from build123d import *

# Parameters (mm, degrees)
BOSS_EXTRUDE1_DEPTH = 64
SKETCH2_R           = 2
CUT_EXTRUDE1_DEPTH  = 5.7
CUT_EXTRUDE2_START  = -5.7
SKETCH3_R           = 2
CUT_EXTRUDE2_DEPTH  = 5.7


with BuildPart() as part:
    # Sketch1 → Boss-Extrude1 (new body)
    with BuildSketch(Plane(origin=(0, 0, 0), x_dir=(1, 0, 0), z_dir=(0, 1, 0))):
        Polygon((-19.5, 39.5), (-19.5, -39.5), (12.5, -39.5), (12.5, -32.5), (-12.5, -32.5), (-12.5, 32.5), (12.5, 32.5), (12.5, 39.5), align=None)
    extrude(amount=BOSS_EXTRUDE1_DEPTH)

    # Sketch2 → Cut-Extrude1 (cut)
    with BuildSketch(Plane(origin=(0, 0, 0), x_dir=(1, 0, 0), z_dir=(0, 1, 0))):
        with Locations(Location((-16, 36, 0), (0, 0, 270))):
            Circle(SKETCH2_R)
        with Locations(Location((-16, -36, 0), (0, 0, 90))):
            Circle(SKETCH2_R)
        with Locations(Location((9, 36, 0), (0, 0, 270))):
            Circle(SKETCH2_R)
        with Locations(Location((9, -36, 0), (0, 0, 90))):
            Circle(SKETCH2_R)
    extrude(amount=CUT_EXTRUDE1_DEPTH, mode=Mode.SUBTRACT)

    # Sketch3 → Cut-Extrude2 (cut)
    with BuildSketch(Plane(origin=(0, 64, 0), x_dir=(1, 0, 0), z_dir=(0, 1, 0)).offset(CUT_EXTRUDE2_START)):
        with Locations(Location((-16, 0, 0), (0, 0, 270))):
            Circle(SKETCH3_R)
        with Locations(Location((9, -36, 0), (0, 0, 90))):
            Circle(SKETCH3_R)
        with Locations(Location((9, 36, 0), (0, 0, 270))):
            Circle(SKETCH3_R)
    extrude(amount=CUT_EXTRUDE2_DEPTH, mode=Mode.SUBTRACT)


solid = part.part
Read the model definition and answer for the solid it produces. Units are mm, in the model's axes. A direction names the side the tool comes from. Round coordinates to 2 decimals unless told otherwise and drop trailing zeros. Order: outer loops, then holes, each group sorted by start corner. A loop starts at its lowest first (then second) coordinate and runs counter-clockwise, first axis right, second up. Notation, with made-up numbers: (73.5, 19.25) - (85.5, 19.25) arc R28 ccw to (85.5, 56.25) - close; hole circle Ø8 at (20, 73). An arc over 180 degrees is marked (long way). Use one line per item in the form item = value. Start each with the question number.
(1) The part is cut by section C-C (z = -36). Give the vertices of the cut face in (x, y).
(2) Find the intervals of material crossed by line 1 along X through (y, z) = (3.5, 36); line 2 along Z through (x, y) = (8.5, 19.5); line 3 along X through (y, z) = (62.8, 0), in increasing order. Write a range as from..to.
(3) Flat-ended cylindrical pins translate along their axes: pin 1 Ø1.5 at (y, z) = (27, 31.5) entering from +X; pin 2 Ø2 at (x, z) = (9, -35.5) entering from +Y; pin 3 Ø3.5 at (x, z) = (9, -36) entering from -Y. Find the tip coordinate at first contact, or state that the pin passes through.
(4) The part is cut by section A-A (x = 9). Give the vertices of the cut face in (y, z), then the cut area to 3 significant figures.
(5) Determine the mould class of faces 5 (the face through (9, 58.3, -36)), 6 (the face through (-19.5, 32, -1)), 7 (the face through (-18, 64, -1)) for opening direction X: +X half, -X half, draft (parallel to the pull), parting line (faces both ways), or undercut.
(6) The part is cut by section B-B (y = 40.5). Give the vertices of the cut face in (x, z).
(7) The part is cut by section D-D (x = -4.5). Give the vertices of the cut face in (y, z).
(8) For faces 1 (the face through (9, 5.7, -36)), 2 (the face through (-12.5, 32, 0)), 3 (the face through (-4, 32, 39.5)), 4 (the face through (-14, 61, 0)), determine the directions among +Z, -Z, +X, -X, +Y, -Y from which every point of the face is accessible in a straight line to the end or side of a thin tool.
Checked values:
q1.outline = (-19.5, 0) - (-18, 0) - (-18, 5.7) - (-14, 5.7) - (-14, 0) - (7, 0) - (7, 5.7) - (11, 5.7) - (11, 0) - (12.5, 0) - (12.5, 64) - (11, 64) - (11, 58.3) - (7, 58.3) - (7, 64) - (-19.5, 64) - close
q2.line_1 = -19.5..-18, -14..7, 11..12.5
q2.line_2 = -39.5..-32.5, 32.5..39.5
q2.line_3 = -19.5..-18, -14..-12.5
q3.pin_1 = -12.5
q3.pin_2 = 58.3
q3.pin_3 = 5.7
q4.outline = (0, -39.5) - (64, -39.5) - (64, -38) - (58.3, -38) - (58.3, -34) - (64, -34) - (64, -32.5) - (0, -32.5) - (0, -34) - (5.7, -34) - (5.7, -38) - (0, -38) - close; (0, 32.5) - (64, 32.5) - (64, 34) - (58.3, 34) - (58.3, 38) - (64, 38) - (64, 39.5) - (0, 39.5) - (0, 38) - (5.7, 38) - (5.7, 34) - (0, 34) - close
q4.area = 805 mm^2
q5.face_5 = undercut
q5.face_6 = -X half
q5.face_7 = draft
q6.outline = (-19.5, -39.5) - (12.5, -39.5) - (12.5, -32.5) - (-12.5, -32.5) - (-12.5, 32.5) - (12.5, 32.5) - (12.5, 39.5) - (-19.5, 39.5) - close
q7.outline = (0, -39.5) - (64, -39.5) - (64, -32.5) - (0, -32.5) - close; (0, 32.5) - (64, 32.5) - (64, 39.5) - (0, 39.5) - close
q8.face_1 = -Y
q8.face_2 = +X, +Y, -Y
q8.face_3 = +Z, +X, -X, +Y, -Y
q8.face_4 = +Y
